```python
from build123d import *

# Parameters (mm, degrees)
SKETCH1_W           = 278.5
SKETCH1_H           = 285
BOSS_EXTRUDE1_DEPTH = 3
SKETCH2_W           = 15
SKETCH2_H           = 1.5
CUT_EXTRUDE1_DEPTH  = 318.213748914
CUT_EXTRUDE3_REACH  = 201.263
SKETCH4_R           = 2.5
CUT_EXTRUDE4_REACH  = 201.263
SKETCH5_R           = 2.5


with BuildPart() as part:
    # Sketch1 → Boss-Extrude1 (new body)
    with BuildSketch(Plane(origin=(0, 0, 0), x_dir=(1, 0, 0), z_dir=(0, 1, 0))):
        Rectangle(SKETCH1_W, SKETCH1_H)
    extrude(amount=BOSS_EXTRUDE1_DEPTH)

    # Sketch2 → Cut-Extrude1 (cut, through all)
    with BuildSketch(Plane.XY.offset(142.5)):
        with Locations((131.75, 2.25)):
            Rectangle(SKETCH2_W, SKETCH2_H)
    extrude(amount=-CUT_EXTRUDE1_DEPTH, mode=Mode.SUBTRACT)

    # Sketch4 → Cut-Extrude3 (cut, up to next)
    with BuildSketch(Plane.XZ, mode=Mode.PRIVATE) as cut_extrude3_sk1:
        with Locations(Location((-109.25, -132.5, 0), (0, 0, 270))):
            Circle(SKETCH4_R)
    cut_extrude3_tool1 = extrude(cut_extrude3_sk1.sketch, amount=-CUT_EXTRUDE3_REACH, mode=Mode.PRIVATE) & part.part
    # Sketch4 → Cut-Extrude3 (cut, up to next)
    with BuildSketch(Plane.XZ, mode=Mode.PRIVATE) as cut_extrude3_sk2:
        with Locations(Location((-109.25, 132.5, 0), (0, 0, 270))):
            Circle(SKETCH4_R)
    cut_extrude3_tool2 = extrude(cut_extrude3_sk2.sketch, amount=-CUT_EXTRUDE3_REACH, mode=Mode.PRIVATE) & part.part
    add(cut_extrude3_tool1.solids().sort_by_distance((-109.25, 0, -132.5))[0], mode=Mode.SUBTRACT)
    add(cut_extrude3_tool2.solids().sort_by_distance((-109.25, 0, 132.5))[0], mode=Mode.SUBTRACT)

    # Sketch5 → Cut-Extrude4 (cut, up to next)
    with BuildSketch(Plane.XZ, mode=Mode.PRIVATE) as cut_extrude4_sk1:
        with Locations(Location((131.75, -112.5, 0), (0, 0, 270))):
            Circle(SKETCH5_R)
    cut_extrude4_tool1 = extrude(cut_extrude4_sk1.sketch, amount=-CUT_EXTRUDE4_REACH, mode=Mode.PRIVATE) & part.part
    # Sketch5 → Cut-Extrude4 (cut, up to next)
    with BuildSketch(Plane.XZ, mode=Mode.PRIVATE) as cut_extrude4_sk2:
        with Locations(Location((131.75, 112.5, 0), (0, 0, 270))):
            Circle(SKETCH5_R)
    cut_extrude4_tool2 = extrude(cut_extrude4_sk2.sketch, amount=-CUT_EXTRUDE4_REACH, mode=Mode.PRIVATE) & part.part
    add(cut_extrude4_tool1.solids().sort_by_distance((131.75, 0, -112.5))[0], mode=Mode.SUBTRACT)
    add(cut_extrude4_tool2.solids().sort_by_distance((131.75, 0, 112.5))[0], mode=Mode.SUBTRACT)


solid = part.part
```
Work out the finished part from the listing and answer in its coordinate system (mm). A direction names the side the tool comes from. Round coordinates to 2 decimals unless told otherwise and drop trailing zeros. Write each loop counter-clockwise with the first axis right and the second up, starting at its lowest first coordinate (ties: lowest second). Pieces come first, ordered by that corner, then holes.
1) A cutting plane is placed at A-A on z = 41. Determine the outline of the cut face in (x, y), and give its area (3 significant figures).
2) A cutting plane is placed at B-B on y = 2.45. Determine the outline of the cut face in (x, z), and give its area (3 significant figures).
3) Flat-ended cylindrical pins translate along their axes: P1, Ø3, axis at x = 131.75, z = 112.5, coming from the +Y side; P2, Ø1.5, axis at y = 2.5, z = 92.5, coming from the +X side. Find the tip coordinate at first contact, or state that the pin passes through.
4) Consider probe 1 along Z at (x, y) = (131.75, 0.55); probe 2 along X at (y, z) = (0.75, 132.5); probe 3 along X at (y, z) = (0.55, -112.5). Determine where each line is inside the solid, lowest interval first.
5) Which of the six approach directions +Z, -Z, +X, -X, +Y, -Y give full straight-line access (tool end or side, diameter ignored) to faces 1 (the face through (132, 1.5, 2)), 2 (the face through (-9, 3, -2))?
Entries:
1. outline: (-139.25, 0) - (139.25, 0) - (139.25, 1.5) - (124.25, 1.5) - (124.25, 3) - (-139.25, 3) - close
1. area: 813 mm2
2. outline: (-139.25, -142.5) - (124.25, -142.5) - (124.25, 142.5) - (-139.25, 142.5) - close; hole circle Ø5 at (-109.25, -132.5); hole circle Ø5 at (-109.25, 132.5)
2. area: 75,100 mm2
3. P1: passes through
3. P2: stops at x = 124.25
4. probe 1: z = -142.5 to -115, -110 to 110, 115 to 142.5
4. probe 2: x = -139.25 to -111.75, -106.75 to 139.25
4. probe 3: x = -139.25 to 129.25, 134.25 to 139.25
5. face 1: +Z, -Z, +X, +Y
5. face 2: +Z, -Z, +X, -X, +Y
